```python
from build123d import *

# Parameters (mm, degrees)
F1_DEPTH = 63.5


with BuildPart() as f1:
    # F0 (on Front) → F1 (new body, symmetric)
    with BuildSketch(Plane.XZ):
        with BuildLine():
            Line((33.02, 38.1), (0, 38.1))
            Line((0, 38.1), (0, 0))
            Line((0, 0), (0, -38.1))
            Line((0, -38.1), (33.02, -38.1))
            ThreePointArc((33.02, -38.1), (35.502395, -36.097882), (34.071366, -33.247808))
            Line((34.071366, -33.247808), (32.724711, -33.037223))
            Line((32.724711, -33.037223), (8.423599, -29.237091))
            ThreePointArc((8.423599, -29.237091), (5.484684, -27.59914), (4.318, -24.44336))
            Line((4.318, -24.44336), (4.318, 0))
            Line((4.318, 0), (4.318, 24.44336))
            ThreePointArc((4.318, 24.44336), (5.484684, 27.59914), (8.423599, 29.237091))
            Line((8.423599, 29.237091), (32.724711, 33.037223))
            Line((32.724711, 33.037223), (34.071366, 33.247808))
            ThreePointArc((34.071366, 33.247808), (35.502395, 36.097882), (33.02, 38.1))
        make_face()
    extrude(amount=F1_DEPTH, both=True)


solid = f1.part
```
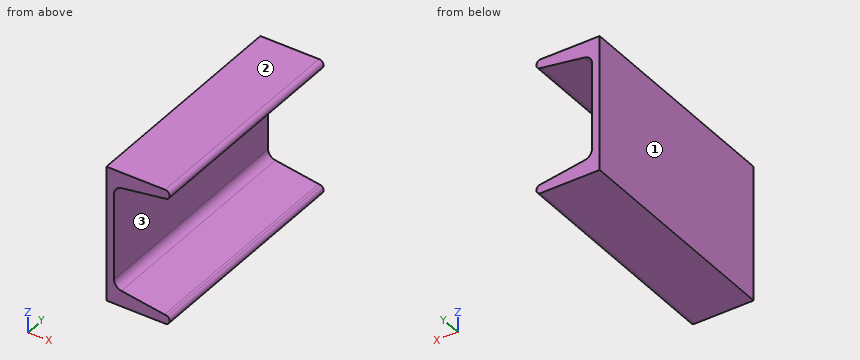
Read the model definition and answer for the solid it produces. Units are mm, in the model's axes. Face numbers are marked on the shaded views. Coordinates: 2 decimals unless noted, no trailing zeros. Write each loop counter-clockwise with the first axis right and the second up, starting at its lowest first coordinate (ties: lowest second). Pieces come first, ordered by that corner, then holes. Notation, with made-up numbers: (87.5, 15) - (143.5, 15) arc R17 ccw to (143.5, 40) - close; hole circle Ø9 at (21, 73). An arc over 180 degrees is marked (long way). Answer as a JSON object with one key per item and string values. Group by question number.
1. A cutting plane is placed at C-C (x = 29). Determine the outline of the cut face in (y, z).
2. A cutting plane is placed at B-B (y = -10.5). Determine the outline of the cut face in (x, z).
3. A cutting plane is placed at D-D (z = -17.5). Determine the outline of the cut face in (x, y), plus the area to 3 significant figures.
4. Consider L1, parallel to X at y = 35, z = 12.5; L2, parallel to Z at x = 29.5, y = -13.5; L3, parallel to Z at x = 11, y = 56. Determine where each line is inside the solid, lowest interval first. Write a range as [from, to].
5. The mould has two halves that part along Z. Classify the marked faces 1, 2 and 3: +Z half, -Z half, draft (parallel to the pull), parting line (faces both ways), or undercut.
6. A cutting plane is placed at A-A (x = 23). Determine the outline of the cut face in (y, z), plus the area to 3 significant figures.
Worked out:
{
 "1": {"outline": "(-63.5, -38.1) - (63.5, -38.1) - (63.5, -32.45) - (-63.5, -32.45) - close; (-63.5, 32.45) - (63.5, 32.45) - (63.5, 38.1) - (-63.5, 38.1) - close"},
 "2": {"outline": "(0, -38.1) - (33.02, -38.1) arc R2.54 ccw to (34.07, -33.25) - (32.72, -33.04) - (8.42, -29.24) arc R4.85 cw to (4.32, -24.44) - (4.32, 24.44) arc R4.85 cw to (8.42, 29.24) - (32.72, 33.04) - (34.07, 33.25) arc R2.54 ccw to (33.02, 38.1) - (0, 38.1) - close"},
 "3": {"outline": "(0, -63.5) - (4.32, -63.5) - (4.32, 63.5) - (0, 63.5) - close", "area": "548 mm²"},
 "4": {"L1": "x = [0, 4.32]", "L2": "z = [-38.1, -32.53], [32.53, 38.1]", "L3": "z = [-38.1, -29.64], [29.64, 38.1]"},
 "5": {"face 1": "draft", "face 2": "+Z half", "face 3": "undercut"},
 "6": {"outline": "(-63.5, -38.1) - (63.5, -38.1) - (63.5, -31.52) - (-63.5, -31.52) - close; (-63.5, 31.52) - (63.5, 31.52) - (63.5, 38.1) - (-63.5, 38.1) - close", "area": "1,670 mm²"}
}
